from build123d import *

# Parameters (mm, degrees)
SKETCH2_W           = 17
SKETCH2_H           = 17.16
BOSS_EXTRUDE1_DEPTH = 25.04
SKETCH3_R           = 1.55
BOSS_EXTRUDE2_DEPTH = 4.9
SKETCH4_R           = 0.75
CUT_EXTRUDE1_DEPTH  = 4.9
SKETCH6_R           = 0.75
CUT_EXTRUDE3_DEPTH  = 4.9
SKETCH7_W           = 17
SKETCH7_H           = 13.52
CUT_EXTRUDE4_DEPTH  = 5.17
CUT_EXTRUDE5_REACH  = 35.132
SKETCH8_W           = 14.67
SKETCH8_H           = 4
SKETCH9_W           = 13.54
SKETCH9_H           = 5.64
CUT_EXTRUDE7_DEPTH  = 15.01
BOSS_EXTRUDE3_DEPTH = 18.46


with BuildPart() as part:
    # Sketch2 → Boss-Extrude1 (new body)
    with BuildSketch(Plane.XY):
        Rectangle(SKETCH2_W, SKETCH2_H)
    extrude(amount=BOSS_EXTRUDE1_DEPTH)

    # Sketch3 → Boss-Extrude2 (add)
    with BuildSketch(Plane(origin=(0, 8.58, 0), x_dir=(1, 0, 0), z_dir=(0, 1, 0))):
        with Locations(Location((3.616285273, -22.901678995, 0), (0, 0, 90))):
            Circle(SKETCH3_R)
        with Locations(Location((-3.446563333, -22.884960512, 0), (0, 0, 90))):
            Circle(SKETCH3_R)
    extrude(amount=BOSS_EXTRUDE2_DEPTH)

    # Sketch4 → Cut-Extrude1 (cut)
    with BuildSketch(Plane(origin=(0, 13.48, 0), x_dir=(1, 0, 0), z_dir=(0, 1, 0))):
        with Locations(Location((3.616285273, -22.901678995, 0), (0, 0, 270))):
            Circle(SKETCH4_R)
    extrude(amount=-CUT_EXTRUDE1_DEPTH, mode=Mode.SUBTRACT)

    # Sketch6 → Cut-Extrude3 (cut)
    with BuildSketch(Plane(origin=(0, 13.48, 0), x_dir=(1, 0, 0), z_dir=(0, 1, 0))):
        with Locations(Location((-3.446563333, -22.884960512, 0), (0, 0, 270))):
            Circle(SKETCH6_R)
    extrude(amount=-CUT_EXTRUDE3_DEPTH, mode=Mode.SUBTRACT)

    # Sketch7 → Cut-Extrude4 (cut)
    with BuildSketch(Plane.XZ.offset(8.58)):
        with Locations((0, 8.21)):
            Rectangle(SKETCH7_W, SKETCH7_H)
    extrude(amount=-CUT_EXTRUDE4_DEPTH, mode=Mode.SUBTRACT)

    # Sketch8 → Cut-Extrude5 (cut, up to next)
    with BuildSketch(Plane.ZY.offset(8.5), mode=Mode.PRIVATE) as cut_extrude5_sk1:
        with Locations((7.335, 6.58)):
            Rectangle(SKETCH8_W, SKETCH8_H)
    cut_extrude5_tool1 = extrude(cut_extrude5_sk1.sketch, amount=-CUT_EXTRUDE5_REACH, mode=Mode.PRIVATE) & part.part
    add(cut_extrude5_tool1.solids().sort_by_distance((-8.5, 6.58, 7.335))[0], mode=Mode.SUBTRACT)

    # Sketch9 → Cut-Extrude7 (cut)
    with BuildSketch(Plane.ZY.offset(8.5)):
        with Locations((8.22, -0.59)):
            Rectangle(SKETCH9_W, SKETCH9_H)
    extrude(amount=-CUT_EXTRUDE7_DEPTH, mode=Mode.SUBTRACT)

    # Sketch10 → Boss-Extrude3 (add)
    with BuildSketch(Plane(origin=(0, 4.58, 0), x_dir=(1, 0, 0), z_dir=(0, 1, 0))):
        with BuildLine():
            Line((5.165, -13.27), (-5.165, -13.27))
            ThreePointArc((-5.165, -13.27), (-7.623357493, -7.335), (-5.165, -1.4))
            Line((-5.165, -1.4), (5.165, -1.4))
            ThreePointArc((5.165, -1.4), (7.623357493, -7.335), (5.165, -13.27))
        make_face()
    extrude(amount=BOSS_EXTRUDE3_DEPTH)


solid = part.part
Check sheet for the modelled part. Datum: model origin and axes. Units: mm. A direction names the side the tool comes from. Round coordinates to 2 decimals unless told otherwise and drop trailing zeros. Loops run counter-clockwise (first coordinate to the right, second up) from the corner with the lowest first, then second, coordinate; pieces in that order, holes last.
1. Sectioned sample at D-D on z = 11. Record the boundary of the cut face in (x, y).
2. Set-up check for faces 1 (the flat face through (0, 14, 1.4)), 2 (the cylindrical face through (4.21, 11, 21.47)), 3 (the flat face through (0, 7, 14.67)), 4 (the flat face through (0, -3, 1.45)): record each of +Z, -Z, +X, -X, +Y, -Y from which the full face is reachable in a straight line by a thin tool's end or side.
3. Scan lines: probe 1 along Z at (x, y) = (-7, -4.5); probe 2 along Z at (x, y) = (-2.25, 7.5); probe 3 along Y at (x, z) = (-6.75, 13.75). Record each from-to range of solid material in increasing order.
4. Mould release check, pull along X, two halves, no side actions. Record for faces 5 (the cylindrical face through (-2.853, 10.996, 21.453)), 6 (the flat face through (8.5, 0, 15)), 7 (the flat face through (3, 13.48, 22)): released by +X, released by -X, zero draft, split by the parting line, or undercut.
5. Gauge pin test, flat ends, axial feed: pin 1 Ø5 at (x, y) = (1, 16.5) entering from -Z; pin 2 Ø2 at (y, z) = (16, 10) entering from +X; pin 3 Ø1.5 at (x, z) = (4, 23.5) entering from +Y; pin 4 Ø5 at (x, z) = (-4.5, 15) entering from +Y. Record the tip position at first contact, or that the pin passes through.
6. Sectioned sample at A-A on y = -4. Record the boundary of the cut face in (x, z).
7. Sectioned sample at B-B on y = 11.5. Record the boundary of the cut face in (x, z) (3 decimals).
Recorded:
1. outline: (-8.5, 2.23) - (6.51, 2.23) - (6.51, -3.41) - (8.5, -3.41) - (8.5, 4.58) - (6.78, 4.58) - (6.78, 23.04) - (-6.78, 23.04) - (-6.78, 4.58) - (-8.5, 4.58) - close
2. face 1: -Z, +X, -X, +Y
2. face 2: +Y
2. face 3: +X, -X, +Y
2. face 4: -X, -Y
3. probe 1: z = 0 to 1.45, 14.97 to 25.04
3. probe 2: z = 1.4 to 13.27, 14.67 to 25.04
3. probe 3: y = 2.23 to 4.58
4. face 5: undercut
4. face 6: released by +X
4. face 7: zero draft
5. pin 1: stops at z = 1.4
5. pin 2: stops at x = 7.46
5. pin 3: stops at y = 13.48
5. pin 4: stops at y = 23.04
6. outline: (-8.5, 0) - (8.5, 0) - (8.5, 1.45) - (-8.5, 1.45) - close; (-8.5, 14.97) - (8.5, 14.97) - (8.5, 25.04) - (-8.5, 25.04) - close
7. outline: (-5.165, 1.4) - (5.165, 1.4) arc R8.393 ccw to (5.165, 13.27) - (-5.165, 13.27) arc R8.393 ccw to start; circle Ø3.1 at (-3.447, 22.885); circle Ø3.1 at (3.616, 22.902); hole circle Ø1.5 at (-3.447, 22.885); hole circle Ø1.5 at (3.616, 22.902)
